```python
from build123d import *

# Parameters (mm, degrees)
SKETCH_1_R      = 6
SKETCH_1_R_2    = 2
EXTRUDE_1_DEPTH = 2
EXTRUDE_START   = -1
SKETCH_2_R      = 6.75
SKETCH_2_R_2    = 2
EXTRUDE_2_DEPTH = 1
CHAMFER_1_SIZE  = 0.2


with BuildPart() as part:
    # 草图1 → 凸台-拉伸1 (new, symmetric)
    with BuildSketch(Plane.XY):
        Circle(SKETCH_1_R)
        Circle(SKETCH_1_R_2, mode=Mode.SUBTRACT)
    extrude(amount=EXTRUDE_1_DEPTH, both=True)

    # 草图2 → 凸台-拉伸2 (add)
    with BuildSketch(Plane.XY.offset(2).offset(EXTRUDE_START)):
        Circle(SKETCH_2_R)
        Circle(SKETCH_2_R_2, mode=Mode.SUBTRACT)
    extrude(amount=EXTRUDE_2_DEPTH)

    # 倒角1
    chamfer_1_edges = [part.edges().sort_by_distance(p)[0] for p in [
        (-6.75, 0, 2),
        (-6.75, 0, 1),
        (-6, 0, -2),
    ]]
    chamfer(chamfer_1_edges, length=CHAMFER_1_SIZE)


solid = part.part
```
Geometry check sheet. Reference: the model listing, model coordinates, mm. A direction names the side the tool comes from. Give positions to 0.01 mm unless a question says otherwise; leave off trailing zeros. Order: outer loops, then holes, each group sorted by start corner. A loop starts at its lowest first (then second) coordinate and runs counter-clockwise, first axis right, second up.
1. Gauge pin test, flat end, axial feed: pin 1 Ø1.5 at (y, z) = (-4.5, 0) entering from -X. Record the tip position at first contact, or that the pin passes through.
2. Release check for a two-part mould opening along X. For faces 1 (the face through (0, -2, 0)), 2 (the face through (1, 2, 2)), 3 (the face through (-6, 0, 0)) record: pulls with the +X half, pulls with the -X half, needs draft (parallel to the pull), parting line crosses it, or undercut.
3. Access from +Z, -Z, +X, -X, +Y, -Y to the whole of each face (thin tool, end or side, straight path). Record for faces 4 (the face through (6, -2, 1)), 5 (the face through (2.5, 0.1, -2)).
4. Section check A-A, the plane y = 0. Enter the section's corners in (x, z).
5. Section check C-C, the plane z = -1.25. Enter the section's corners in (x, y).
6. Thickness scan on L1, parallel to Y at x = 0, z = -1.1; L2, parallel to Y at x = -1.25, z = -1.4; L3, parallel to Z at x = -4, y = -4.75. Record the ranges inside material, lowest first.
Values follow:
1. pin 1: stops at x = -4.68
2. face 1: undercut
2. face 2: needs draft
2. face 3: parting line crosses it
3. face 4: -Z
3. face 5: -Z, +X, -X, +Y, -Y
4. outline: (-6.75, 1.2) - (-6.55, 1) - (-6, 1) - (-6, -1.8) - (-5.8, -2) - (-2, -2) - (-2, 2) - (-6.55, 2) - (-6.75, 1.8) - close; (2, -2) - (5.8, -2) - (6, -1.8) - (6, 1) - (6.55, 1) - (6.75, 1.2) - (6.75, 1.8) - (6.55, 2) - (2, 2) - close
5. outline: circle Ø12 at (0, 0); hole circle Ø4 at (0, 0)
6. L1: y = -6 to -2, 2 to 6
6. L2: y = -5.87 to -1.56, 1.56 to 5.87
6. L3: z = 1 to 2
